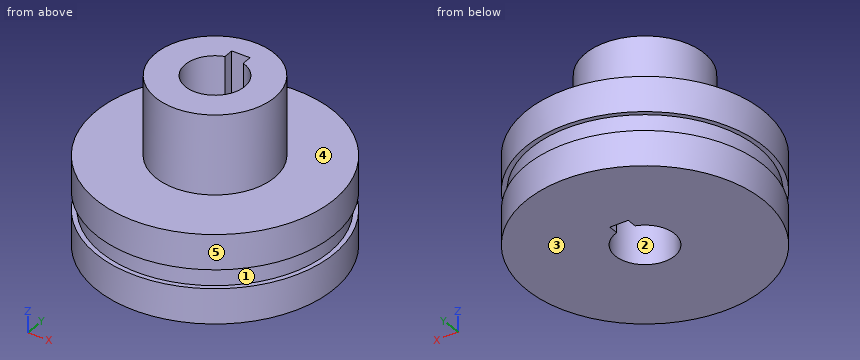
Autodesk Inventor part; units mm, degrees
ref_plane "YZ Plane" through (0, 0, 0) normal (1, 0, 0) x (0, 1, 0)
ref_plane "XZ Plane" through (0, 0, 0) normal (0, 1, 0) x (-1, 0, 0)
ref_plane "XY Plane" through (0, 0, 0) normal (0, 0, 1) x (1, 0, 0)
sketch "Sketch4" plane through (0, 0, 0) normal (0, 0, 1) x (1, 0, 0)
  circle A0 centre (0, 0) radius 18.3
  dimension "d9" = 36.6
extrude "Extrusion4" add sketch "Sketch4" along normal blind 3
sketch "Sketch5" plane through (0, 0, 3) normal (0, 0, 1) x (1, 0, 0)
  circle A0 centre (0, 0) radius 18.3
  circle A1 centre (0, 0) radius 19.05
  dimension "d12" = 38.1
extrude "Extrusion5" add sketch "Sketch5" along normal blind 5.6 contours A0 | A1
sketch "Sketch6" plane through (0, 0, 0) normal (0, 0, -1) x (-1, 0, 0)
  circle A0 centre (0, 0) radius 18.3
  circle A1 centre (0, 0) radius 19.05
  dimension "d15" = 38.1
extrude "Extrusion6" add sketch "Sketch6" along normal blind 5.6 contours A0 | A1
sketch "Sketch7" plane through (0, 0, 8.6) normal (0, 0, 1) x (1, 0, 0)
  circle A0 centre (0, 0) radius 19.05
  circle A1 centre (0, 0) radius 9.525
  dimension "d18" = 19.05
extrude "Extrusion7" add sketch "Sketch7" along normal blind 12.7 contours A1
sketch "Sketch8" plane through (0, 0, -5.6) normal (0, 0, -1) x (-1, 0, 0)
  circle A0 centre (0, 0) radius 19.05
  circle A1 centre (0, 0) radius 4.7625
  dimension "d21" = 9.525
extrude "Extrusion8" cut sketch "Sketch8" against normal blind 38.1 contours A1
sketch "Sketch9" plane through (0, 0, -5.6) normal (0, 0, -1) x (-1, 0, 0)
  circle A0 centre (0, 0) radius 4.7625
  line L0 (-1.4638, 3.2131) -> (1.4638, 3.2131)
  line L1 (1.4638, 3.2131) -> (1.4638, 6.1406)
  line L2 (1.4638, 6.1406) -> (-1.4638, 6.1406)
  line L3 (-1.4638, 6.1406) -> (-1.4638, 3.2131)
  dimension "d24" = 2.9276
  dimension "d25" = 2.9276
  dimension "d26" = 3.2131
  dimension "d27" = 1.4638
extrude "Extrusion9" cut sketch "Sketch9" against normal blind 38.1 contours L1 L0 L3 A0 | A0 L3 L2 L1 picked at (0.165, 3.721)
equation "\"d25\" = d24"
equation "\"d27\" = 0.5 * d25"
properties part number "Puller Wheel"
The listing builds one solid part. Answer for the finished solid, in the listing's coordinates (mm). Face numbers are marked on the shaded views. A direction names the side the tool comes from. Coordinates: 2 decimals unless noted, no trailing zeros. Loops run counter-clockwise (first coordinate to the right, second up) from the corner with the lowest first, then second, coordinate; pieces in that order, holes last. Notation, with made-up numbers: M -32.5,11.5 L -27.5,11.5 A6 cw -27.5,16.5 Z; hole C 71,74.25 d4. An arc over 180 degrees is marked long. Answer in a Markdown table with one row per item.
1) Given pin 1 (1.5 mm diameter, centred on y = 11.5, z = -3, fed in from -X); pin 2 (12 mm diameter, centred on y = -10, z = 17.5, fed in from -X); pin 3 (5 mm diameter, centred on x = -3, z = 15.5, fed in from -Y), each flat-ended and moving along its own axis, determine where each tip first touches the part or whether it passes through.
Answers below:
| item | result |
|---|---|
| pin 1 | x = -15.73 |
| pin 2 | x = -8.64 |
| pin 3 | y = -9.51 |
2) Find section C-C (y = 0.5). Determine the outline of the cut face in (x, z).
Answers below:
| item | result |
|---|---|
| outline | M -19.04,-5.6 L -4.74,-5.6 L -4.74,21.3 L -9.51,21.3 L -9.51,8.6 L -19.04,8.6 L -19.04,3 L -18.29,3 L -18.29,0 L -19.04,0 Z; M 4.74,-5.6 L 19.04,-5.6 L 19.04,0 L 18.29,0 L 18.29,3 L 19.04,3 L 19.04,8.6 L 9.51,8.6 L 9.51,21.3 L 4.74,21.3 Z |
3) Find section D-D (y = -11). Determine the outline of the cut face in (x, z), then the cut area to 3 significant figures.
Answers below:
| item | result |
|---|---|
| outline | M -15.55,-5.6 L 15.55,-5.6 L 15.55,0 L 14.62,0 L 14.62,3 L 15.55,3 L 15.55,8.6 L -15.55,8.6 L -15.55,3 L -14.62,3 L -14.62,0 L -15.55,0 Z |
| area | 436 mm^2 |
4) Determine the mould class of the marked faces 1, 2 and 3 for opening direction X: released by +X, released by -X, zero draft, split by the parting line, or undercut.
Answers below:
| item | result |
|---|---|
| face 1 | split by the parting line |
| face 2 | undercut |
| face 3 | zero draft |
5) Which of the six approach directions +Z, -Z, +X, -X, +Y, -Y give full straight-line access (tool end or side, diameter ignored) to the marked faces 4 and 5?
Answers below:
| item | result |
|---|---|
| face 4 | +Z |
| face 5 | +Z, -Z |
6) Find the intervals of material crossed by probe 1 along Y at (x, z) = (0, 4); probe 2 along Y at (x, z) = (0, 2); probe 3 along Z at (x, y) = (-7.5, 15), in increasing order.
Answers below:
| item | result |
|---|---|
| probe 1 | -19.05 to -4.76, 6.14 to 19.05 |
| probe 2 | -18.3 to -4.76, 6.14 to 18.3 |
| probe 3 | -5.6 to 8.6 |
